Job drawing, mm, ordinate dimensions from the low corner. One solid piece. Give positions to 0.01 mm unless a question says otherwise; leave off trailing zeros. Order: outer loops, then holes, each group sorted by start corner. A loop starts at its lowest first (then second) coordinate and runs counter-clockwise, first axis right, second up. Notation, with made-up numbers: (-13.5, 81) - (10.5, 81) arc R13 ccw to (10.5, 89) - close; hole circle Ø7 at (-15.5, -26). An arc over 180 degrees is marked (long way). Use one line per item in the form item = value. Start each with the question number.
1. Band-saw the part on A-A, the plane x = 62. List the corners of the cut face in (y, z), plus the area to 3 significant figures.
2. Drill centre lines: line 1 (X direction, y = 52, z = 0.5); line 2 (Y direction, x = 62, z = 0.35); line 3 (Y direction, x = 3.5, z = 0.5). Where is each one in solid material? Low to high.
3. Band-saw the part on B-B, the plane y = 52. List the corners of the cut face in (x, z), plus the area to 3 significant figures.
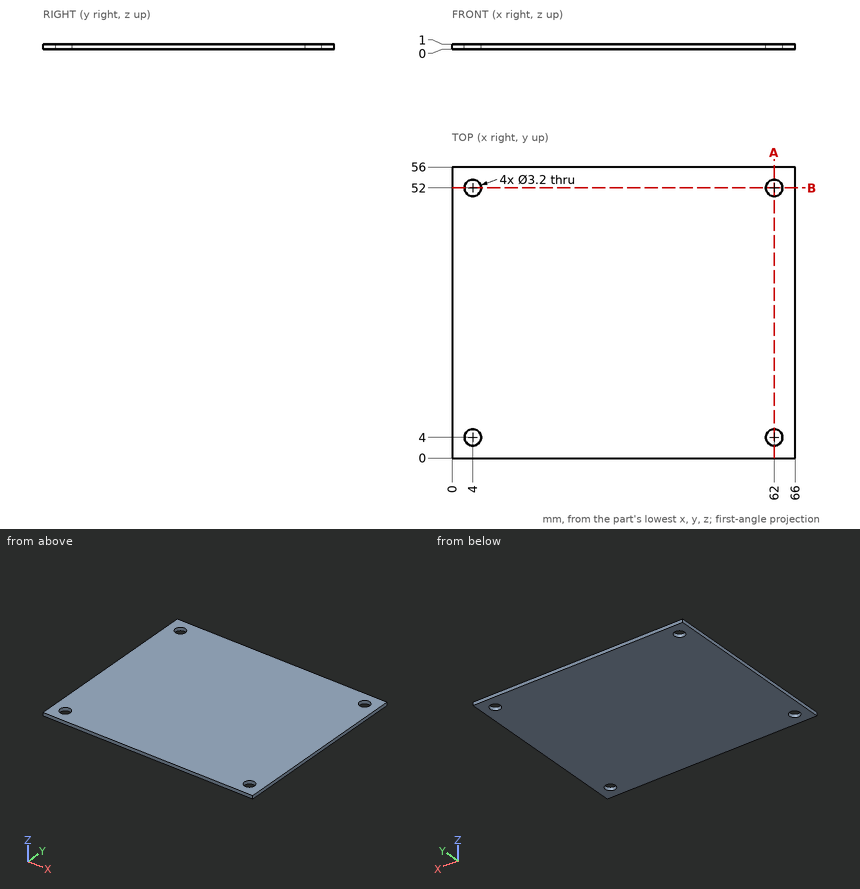
From the geometry:
q1.outline = (0, 0) - (2.4, 0) - (2.4, 1) - (0, 1) - close; (5.6, 0) - (50.4, 0) - (50.4, 1) - (5.6, 1) - close; (53.6, 0) - (56, 0) - (56, 1) - (53.6, 1) - close
q1.area = 49.6 mm²
q2.line_1 = 0 to 2.4, 5.6 to 60.4, 63.6 to 66
q2.line_2 = 0 to 2.4, 5.6 to 50.4, 53.6 to 56
q2.line_3 = 0 to 2.48, 5.52 to 50.48, 53.52 to 56
q3.outline = (0, 0) - (2.4, 0) - (2.4, 1) - (0, 1) - close; (5.6, 0) - (60.4, 0) - (60.4, 1) - (5.6, 1) - close; (63.6, 0) - (66, 0) - (66, 1) - (63.6, 1) - close
q3.area = 59.6 mm²
